Geometry: see drawing. Coordinates: mm, zero at the bounding-box minimum. Coordinates: 2 decimals unless noted, no trailing zeros. Order: outer loops, then holes, each group sorted by start corner. A loop starts at its lowest first (then second) coordinate and runs counter-clockwise, first axis right, second up.
Item 1: Contact query for flat-ended pins moving along their axis: P1, Ø5, axis at x = 6.5, z = 2.5, coming from the -Y side (3 decimals); P2, Ø3, axis at x = 3.5, y = 205, coming from the +Z side (3 decimals); P3, Ø5, axis at x = 3, y = 146, coming from the -Z side (3 decimals). Output: stop coordinate, or through.
Item 2: Section B-B on z = 23.5. Return the cut outline in (x, y) (3 decimals).
Item 3: Ray query, line 1 (Z direction, x = 5, y = 202.5) (3 decimals); line 2 (Z direction, x = 6.5, y = 166.5) (3 decimals); line 3 (Y direction, x = 5.75, z = 112) (3 decimals). Return the intervals inside material, ascending.
Item 4: Section C-C on x = 1.5. State how many separate pieces and enclosed holes the cut face has, then the cut area to 3 significant figures.
Item 5: Section A-A on y = 155. Return the cut outline in (x, z) (3 decimals), then the cut area to 3 significant figures.
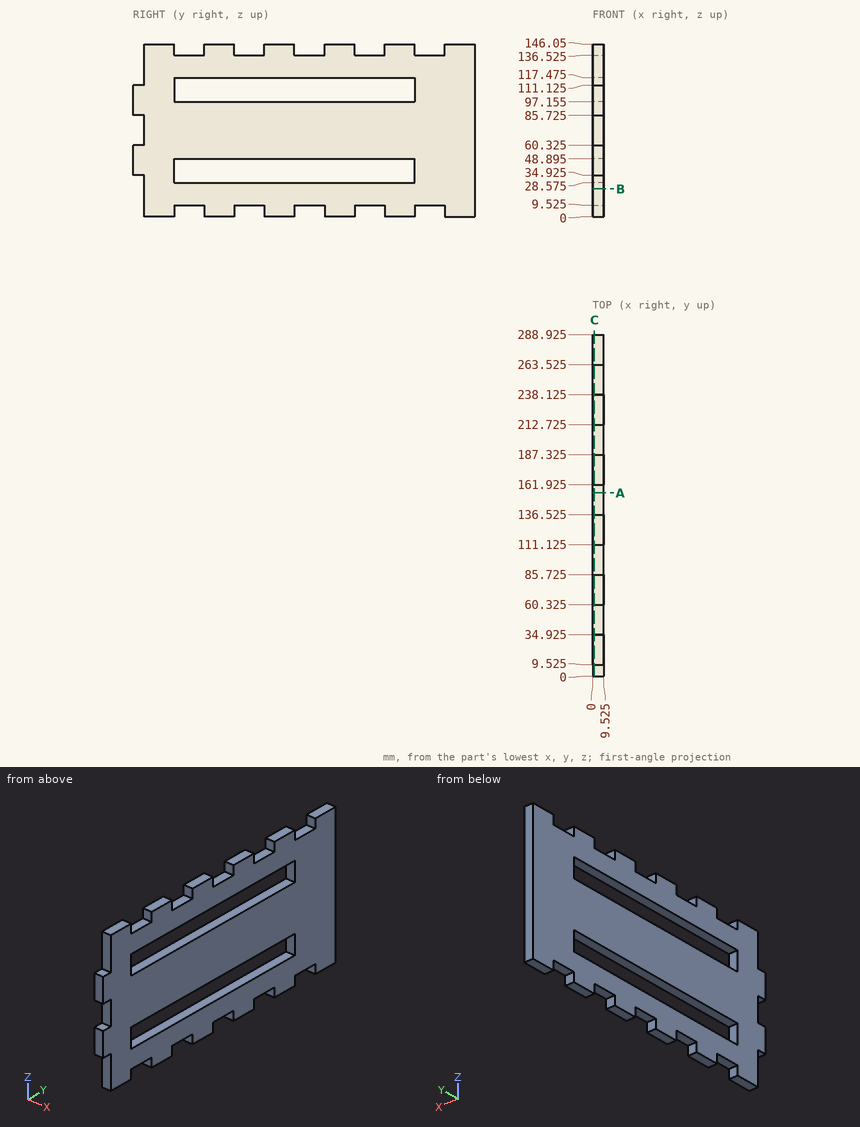
Answer list:
1. P1: stops at y = 9.525
1. P2: stops at z = 136.525
1. P3: stops at z = 9.525
2. outline: (0, 9.525) - (9.525, 9.525) - (9.525, 288.925) - (0, 288.925) - close
3. line 1: z = 9.525 to 28.575, 48.895 to 97.155, 117.475 to 136.525
3. line 2: z = 0 to 28.575, 48.895 to 97.155, 117.475 to 146.05
3. line 3: y = 9.525 to 34.925, 238.125 to 288.925
4. separate pieces: 1
4. enclosed holes: 2
4. area: 30,600 mm2
5. outline: (0, 9.525) - (9.525, 9.525) - (9.525, 28.575) - (0, 28.575) - close; (0, 48.895) - (9.525, 48.895) - (9.525, 97.155) - (0, 97.155) - close; (0, 117.475) - (9.525, 117.475) - (9.525, 136.525) - (0, 136.525) - close
5. area: 823 mm2
